Print and shaded views of the part. All mm, measured from the part's lowest x, y and z. Give positions to 0.01 mm unless a question says otherwise; leave off trailing zeros. Write each loop counter-clockwise with the first axis right and the second up, starting at its lowest first coordinate (ties: lowest second). Pieces come first, ordered by that corner, then holes. Notation, with made-up numbers: M -9.5,36.25 L 19.5,36.25 A10 cw 19.5,47.25 Z; hole C 6.5,21.5 d7. An arc over 180 degrees is marked long. One line per question, with ' | ' between items. Start each with the question number.
1. Cut at B-B, the plane x = 115. Write the cut outline in (y, z).
2. Cut at A-A, the plane y = 5. Write the cut outline in (x, z), then the cut area to 3 significant figures.
3. Wall check: L1, parallel to Y at x = 5, z = 0.6; L2, parallel to X at y = 5, z = 1.4. Give the ranges that are in metal, low to high.
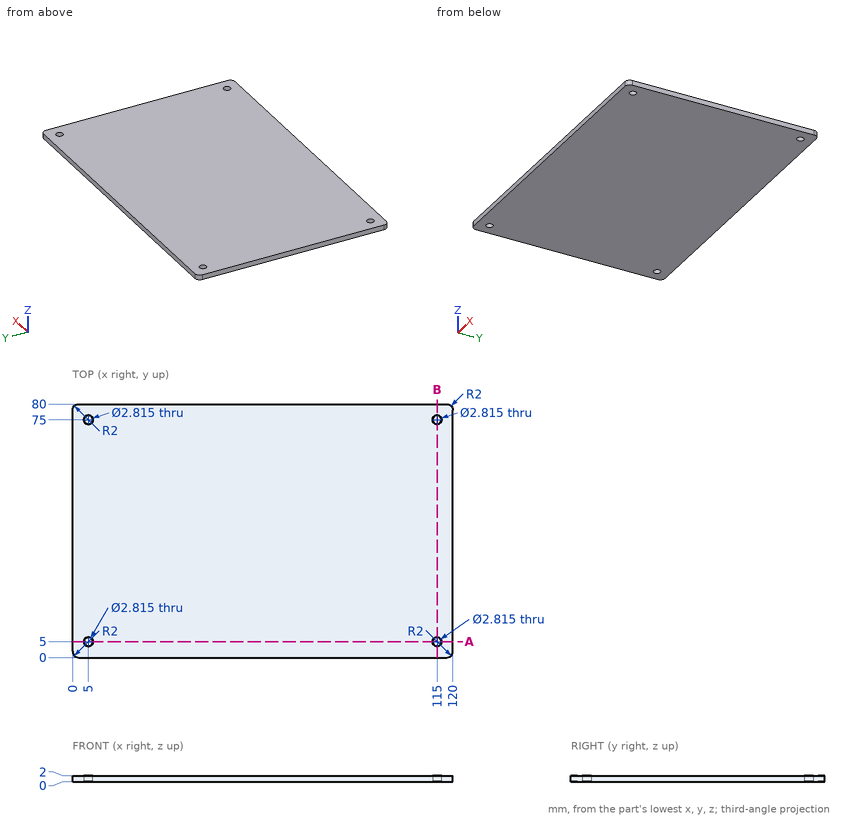
Here are the results:
1) outline: M 0,0 L 3.59,0 L 3.59,2 L 0,2 Z; M 6.41,0 L 73.59,0 L 73.59,2 L 6.41,2 Z; M 76.41,0 L 80,0 L 80,2 L 76.41,2 Z
2) outline: M 0,0 L 3.59,0 L 3.59,2 L 0,2 Z; M 6.41,0 L 113.59,0 L 113.59,2 L 6.41,2 Z; M 116.41,0 L 120,0 L 120,2 L 116.41,2 Z | area: 229 mm^2
3) L1: 0 to 3.59, 6.41 to 73.59, 76.41 to 80 | L2: 0 to 3.59, 6.41 to 113.59, 116.41 to 120
